Here's how the part is built. I have some questions about the finished solid (model axes, mm). Face numbers are marked on the shaded views. A direction names the side the tool comes from. Coordinates: 2 decimals unless noted, no trailing zeros. Write each loop counter-clockwise with the first axis right and the second up, starting at its lowest first coordinate (ties: lowest second). Pieces come first, ordered by that corner, then holes.
Item 1: For the marked faces 1 and 2, which set-ups out of +Z, -Z, +X, -X, +Y, -Y let a thin tool reach every point of the face, with its end or its side?
Item 2: I'm going to push a flat-ended pin straight in: P1, Ø2, axis at x = -348.5, y = -30.5, coming from the +Z side. Where does the tip first touch, or does it pass through?
Item 3: I want a section at A-A (y = 84). Please give me the cut outline in (x, z).
Item 4: I want a section at B-B (z = 211). Please give me the cut outline in (x, y), and give its area (3 significant figures).
Item 5: I want a section at C-C (x = -76.5). Please give me the cut outline in (y, z).
Item 6: If we mould it in two halves opening along Y, with no side actions, what happens to the marked faces 3, 4 and 5? For each: pulls with the +Y half, pulls with the -Y half, needs draft (parallel to the pull), parting line crosses it, or undercut.
Item 7: Please list where these lines run through material, in increasing order: line 1 (Y direction, x = 386, z = 65); line 2 (X direction, y = 68, z = 85.5); line 3 (Z direction, x = -123, y = 109).
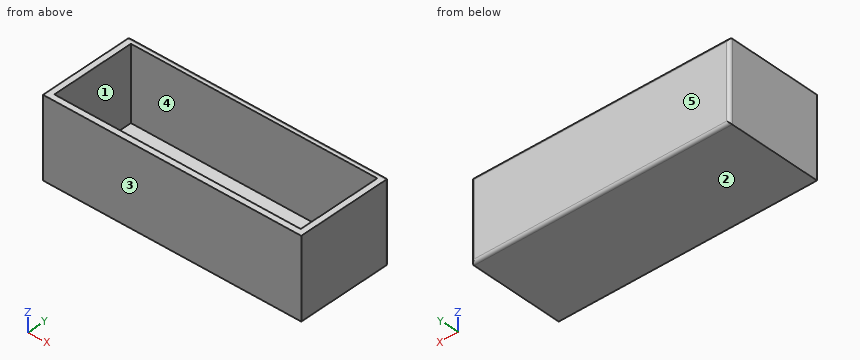
from build123d import *

# Parameters (mm, degrees)
F0_W     = 956
F0_H     = 356
F1_DEPTH = 294
F2_T     = -22
F3_R     = 11


with BuildPart() as f1:
    # F0 (on Top) → F1 (new body)
    with BuildSketch(Plane.XY):
        Rectangle(F0_W, F0_H)
    extrude(amount=F1_DEPTH)

    # F2
    f2_openings = [f1.faces().sort_by_distance(p)[0] for p in [
        (0, 0, 294),
    ]]
    offset(amount=F2_T, openings=f2_openings)

    # F3
    f3_edges = [f1.edges().sort_by_distance(p)[0] for p in [
        (478, 178, 147),
        (-478, 178, 147),
        (0, 178, 0),
        (0, 178, 294),
    ]]
    fillet(f3_edges, radius=F3_R)


solid = f1.part
Answer:
1. face 1: +Z
1. face 2: -Z, +X, -X, +Y, -Y
2. P1: stops at z = 22
3. outline: (-478, 0) - (478, 0) - (478, 294) - (456, 294) - (456, 22) - (-456, 22) - (-456, 294) - (-478, 294) - close
4. outline: (-478, -178) - (478, -178) - (478, 167) arc R11 ccw to (467, 178) - (-467, 178) arc R11 ccw to (-478, 167) - close; hole (-456, -156) - (456, -156) - (456, 156) - (-456, 156) - close
4. area: 55,700 mm2
5. outline: (-178, 0) - (167, 0) arc R11 ccw to (178, 11) - (178, 283) arc R11 ccw to (167, 294) - (156, 294) - (156, 22) - (-156, 22) - (-156, 294) - (-178, 294) - close
6. face 3: pulls with the -Y half
6. face 4: undercut
6. face 5: pulls with the +Y half
7. line 1: y = -178 to -156, 156 to 178
7. line 2: x = -478 to -456, 456 to 478
7. line 3: z = 0 to 22
